```python
from build123d import *

# Parameters (mm, degrees)
SKETCH1_W           = 61.5
SKETCH1_H           = 14
BOSS_EXTRUDE1_DEPTH = 6
SKETCH2_R           = 1.55
CUT_EXTRUDE1_DEPTH  = 64.358109189
SKETCH3_W           = 10
SKETCH3_H           = 14
BOSS_EXTRUDE2_DEPTH = 20
SKETCH4_R           = 1.65
CUT_EXTRUDE2_DEPTH  = 67.168345906
FILLET1_R           = 5


with BuildPart() as part:
    # Sketch1 → Boss-Extrude1 (new body)
    with BuildSketch(Plane(origin=(0, 0, 0), x_dir=(1, 0, 0), z_dir=(0, 1, 0))):
        with Locations((30.75, -7)):
            Rectangle(SKETCH1_W, SKETCH1_H)
    extrude(amount=BOSS_EXTRUDE1_DEPTH)

    # Sketch2 → Cut-Extrude1 (cut, through all)
    with BuildSketch(Plane(origin=(0, 6, 0), x_dir=(1, 0, 0), z_dir=(0, 1, 0))):
        with Locations(Location((19, -4, 0), (0, 0, 270))):
            Circle(SKETCH2_R)
        with Locations(Location((42.5, -4, 0), (0, 0, 270))):
            Circle(SKETCH2_R)
        with Locations(Location((19, -10, 0), (0, 0, 270))):
            Circle(SKETCH2_R)
        with Locations(Location((42.5, -10, 0), (0, 0, 270))):
            Circle(SKETCH2_R)
    extrude(amount=-CUT_EXTRUDE1_DEPTH, mode=Mode.SUBTRACT)

    # Sketch3 → Boss-Extrude2 (add)
    with BuildSketch(Plane(origin=(0, 0, 0), x_dir=(-1, 0, 0), z_dir=(0, -1, 0))):
        with Locations((-5, -7)):
            Rectangle(SKETCH3_W, SKETCH3_H)
        with Locations((-56.5, -7)):
            Rectangle(SKETCH3_W, SKETCH3_H)
    extrude(amount=BOSS_EXTRUDE2_DEPTH)

    # Sketch4 → Cut-Extrude2 (cut, through all)
    with BuildSketch(Plane(origin=(0, 0, 0), x_dir=(-1, 0, 0), z_dir=(0, 0, -1))):
        with Locations((-5, -15)):
            Circle(SKETCH4_R)
        with Locations((-56.5, -15)):
            Circle(SKETCH4_R)
    extrude(amount=-CUT_EXTRUDE2_DEPTH, mode=Mode.SUBTRACT)

    # Fillet1
    fillet1_edges = [part.edges().sort_by_distance(p)[0] for p in [
        (10, -20, 7),
        (0, -20, 7),
        (51.5, -20, 7),
        (61.5, -20, 7),
    ]]
    fillet(fillet1_edges, radius=FILLET1_R - 0.0001)  # a hair under: the kernel refuses the full size


solid = part.part
```
Work out the finished part from the listing and answer in its coordinate system (mm). A direction names the side the tool comes from. Round coordinates to 2 decimals unless told otherwise and drop trailing zeros. Loops run counter-clockwise (first coordinate to the right, second up) from the corner with the lowest first, then second, coordinate; pieces in that order, holes last. Notation, with made-up numbers: (27, -29) -> (71, -29) arc R13 cw to (71, -22) -> close; hole circle Ø9 at (20.25, 31). An arc over 180 degrees is marked (long way). Write each question's results on one line, items separated by ' | '. Start each with the question number.
1. Find the intervals of material crossed by probe 1 along X at (y, z) = (2.6, 10); probe 2 along X at (y, z) = (-6.5, 2); probe 3 along Y at (x, z) = (56.5, 6.5), in increasing order. Write a range as from..to.
2. Section C-C (y = -1.5) is taken. Determine the outline of the cut face in (x, z), plus the area to 3 significant figures.
3. Given pin 1 Ø4 at (x, z) = (42.5, 10) entering from -Y, flat-ended and moving along its own axis, determine where the tip first touches the part or whether it passes through.
4. Section A-A (z = 10) is taken. State how many separate pieces and enclosed holes the cut face has, plus the area to 3 significant figures.
5. Section B-B (x = 19) is taken. Determine the outline of the cut face in (y, z).
6. A tool of negligible diameter and unlimited length cuts with its end or side. For faces 4 (the face through (9, -18, 7)), 5 (the face through (2, -19, 7)), from which of +Z, -Z, +X, -X, +Y, -Y can it reach the whole face along a straight path? Write none if from no direction.
7. For a pull along Y with two mould halves and no side action, classify faces 1 (the face through (60, -18.57, 6.9)), 2 (the face through (38, 2, 0)), 3 (the face through (58.15, -14.93, 6.9)) as +Y half, -Y half, draft (parallel to the pull), parting line (faces both ways), or undercut.
Evaluation:
1) probe 1: x = 0..17.45, 20.55..40.95, 44.05..61.5 | probe 2: x = 0..10, 51.5..61.5 | probe 3: y = -20..-16.65, -13.35..6
2) outline: (0, 0) -> (10, 0) -> (10, 14) -> (0, 14) -> close; (51.5, 0) -> (61.5, 0) -> (61.5, 14) -> (51.5, 14) -> close | area: 280 mm2
3) pin 1: stops at y = 0
4) separate pieces: 3 | enclosed holes: 2 | area: 693 mm2
5) outline: (0, 0) -> (6, 0) -> (6, 2.45) -> (0, 2.45) -> close; (0, 5.55) -> (6, 5.55) -> (6, 8.45) -> (0, 8.45) -> close; (0, 11.55) -> (6, 11.55) -> (6, 14) -> (0, 14) -> close
6) face 4: +Z, -Z, -Y | face 5: +Z, -Z, -X, -Y
7) face 1: -Y half | face 2: draft | face 3: undercut
